Could you check a few things on this drawing? It's one solid part, dimensions in mm from its lowest x, y, z. A direction names the side the tool comes from. Give positions to 0.01 mm unless a question says otherwise; leave off trailing zeros. Order: outer loops, then holes, each group sorted by start corner. A loop starts at its lowest first (then second) coordinate and runs counter-clockwise, first axis right, second up.
(1) Imagine slicing it at B-B, the plane x = 38. Write out the boundary of the cut face in (y, z) (3 decimals), then the cut area to 3 significant figures.
(2) Imagine slicing it at C-C, the plane y = 30. Write out the boundary of the cut face in (x, z), then the cut area to 3 significant figures.
(3) If I drill on probe 1 along X at (y, z) = (5.25, 30.9); probe 2 along Z at (x, y) = (7.5, 2.5); probe 3 along Y at (x, z) = (38, 9) (3 decimals), over which ranges is the centre line in solid material (lowest first)?
(4) Will these pins go through, and if not, where does the flat tip stop? pin 1 (12 mm diameter, centred on y = 16, z = 7.5, fed in from +X); pin 2 (3 mm diameter, centred on x = 12.5, z = 9.5, fed in from +Y) (3 decimals); pin 3 (1.5 mm diameter, centred on y = 10, z = 15.5, fed in from -X).
(5) Imagine slicing it at A-A, the plane z = 10. Write out the boundary of the cut face in (x, y) (3 decimals).
(6) On a 3-axis mill with a long thin cutter (end or side, diameter ignored), from which of +Z, -Z, +X, -X, +Y, -Y can I reach the whole of each face in a straight line? I mean the marked faces 1, 2 and 3. Say none if no direction works.
(7) If we mould it in two halves opening along Y, with no side actions, what happens to the marked faces 4, 5 and 6? For each: released by +Y, released by -Y, zero draft, split by the parting line, or undercut.
(8) Imagine slicing it at D-D, the plane y = 43. Write out the boundary of the cut face in (x, z), then the cut area to 3 significant figures.
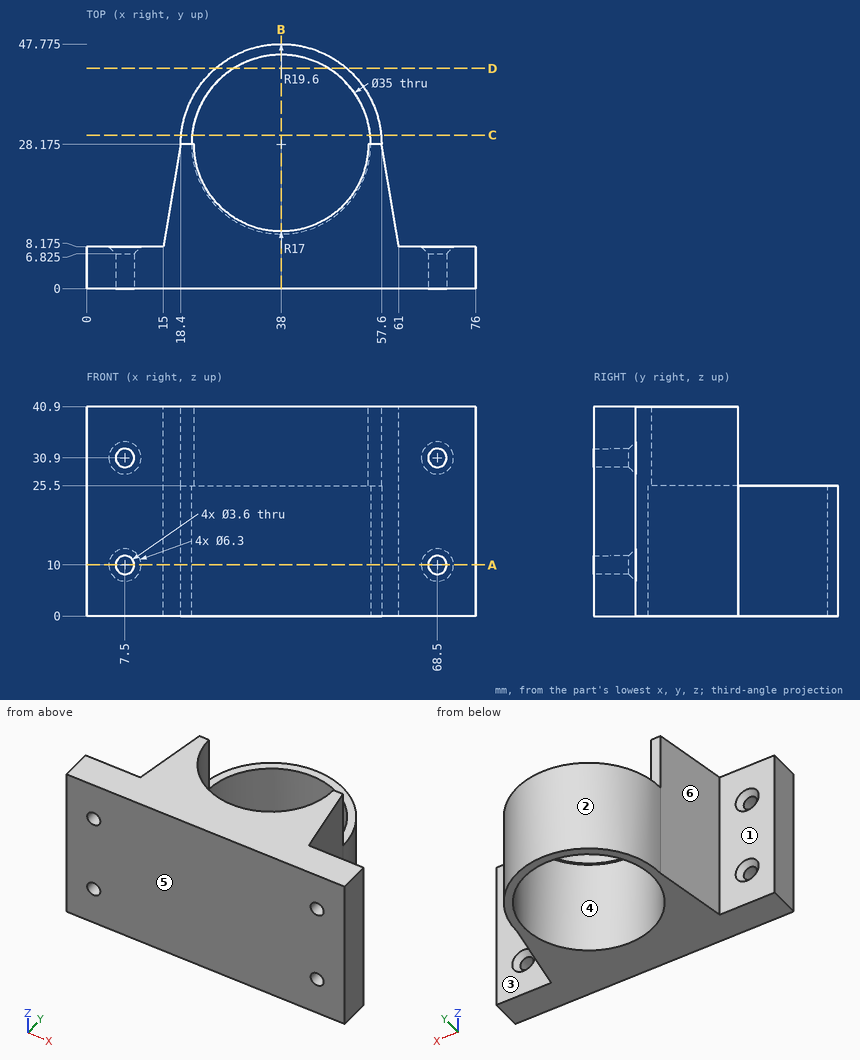
Answer block:
1. outline: (0, 0) - (10.675, 0) - (10.675, 25.5) - (11.175, 25.5) - (11.175, 40.9) - (0, 40.9) - close; (45.675, 0) - (47.775, 0) - (47.775, 25.5) - (45.675, 25.5) - close
1. area: 498 mm2
2. outline: (18.49, 0) - (20.6, 0) - (20.6, 25.5) - (18.49, 25.5) - close; (55.4, 0) - (57.51, 0) - (57.51, 25.5) - (55.4, 25.5) - close
2. area: 108 mm2
3. probe 1: x = 0 to 5.7, 9.3 to 66.7, 70.3 to 76
3. probe 2: z = 0 to 8.2, 11.8 to 29.1, 32.7 to 40.9
3. probe 3: y = 0 to 10.675, 45.675 to 47.775
4. pin 1: stops at x = 60.69
4. pin 2: stops at y = 8.175
4. pin 3: stops at x = 15.18
5. outline: (0, 0) - (5.7, 0) - (5.7, 6.825) - (4.35, 8.175) - (0, 8.175) - close; (9.3, 0) - (66.7, 0) - (66.7, 6.825) - (65.35, 8.175) - (61, 8.175) - (57.6, 28.175) arc R19.6 ccw to (18.4, 28.175) - (15, 8.175) - (10.65, 8.175) - (9.3, 6.825) - close; (70.3, 0) - (76, 0) - (76, 8.175) - (71.65, 8.175) - (70.3, 6.825) - close; hole circle Ø35 at (38, 28.175)
6. face 1: +Z, -Z, -X, +Y
6. face 2: +Z, -Z, +Y
6. face 3: +Z, -Z, +X, +Y
7. face 4: undercut
7. face 5: released by -Y
7. face 6: released by +Y
8. outline: (25.18, 0) - (28.7, 0) - (28.7, 25.5) - (25.18, 25.5) - close; (47.3, 0) - (50.82, 0) - (50.82, 25.5) - (47.3, 25.5) - close
8. area: 180 mm2
